```python
from build123d import *

# Parameters (mm, degrees)
SKETCH5_W                        = 20
SKETCH5_H                        = 45.5
SKETCH5_R                        = 0.55
ULTRASONIC_TRANSDUCER_BASE_DEPTH = 11
ULTRASONIC_PINS_CUTAWAY_DEPTH    = 3
STANDOFF_PROFILE_R               = 1.35
ULTRASONIC_STANDOFFS_DEPTH       = 2
ENCLOSURE_OUTER_LIMIT_W          = 158.6
ENCLOSURE_OUTER_LIMIT_H          = 63.3
ENCLOSURE_BASE_DEPTH             = 1.6
ENCLOSURE_FILLET_R               = 10
SKETCH9_R                        = 2.5
SKETCH9_R_2                      = 3
SKETCH9_R_3                      = 2
UNO_STANDOFFS_DEPTH              = 5.5
UNO_START                        = 1
SKETCH11_R                       = 1.5
UNO_STANDOFF_SCREW_HOLES_DEPTH   = 4.5
ENCLOSURE_WALL_DEPTH             = 27
ENCLOSURE_WALL_DEPTH_BACK        = 1.6
SKETCH13_R                       = 4
LED_RING_CABLE_HOLE_DEPTH        = 1.6
SKETCH14_R                       = 4
BUS_SCREW_POSTS_DEPTH            = 8
SKETCH15_R                       = 1.5
BUS_SCREW_HOLES_DEPTH            = 6
SKETCH16_R                       = 2
POWER_CORD_HOLE_DEPTH            = 1.6
FILLET1_R                        = 1.5
SKETCH6_R                        = 0.6
CUT_PIN_HOLES_DEPTH              = 10


with BuildPart() as part:
    # Sketch5 → Ultrasonic Transducer Base (new body)
    with BuildSketch(Plane(origin=(0, 0, 0), x_dir=(1, 0, 0), z_dir=(0, 1, 0))):
        with Locations((70, 1)):
            Rectangle(SKETCH5_W, SKETCH5_H)
        with Locations((61.4, 22.35)):
            Circle(SKETCH5_R, mode=Mode.SUBTRACT)
        with Locations((78.6, 22.35)):
            Circle(SKETCH5_R, mode=Mode.SUBTRACT)
        with Locations((78.6, -20.35)):
            Circle(SKETCH5_R, mode=Mode.SUBTRACT)
        with Locations((61.4, -20.35)):
            Circle(SKETCH5_R, mode=Mode.SUBTRACT)
    extrude(amount=ULTRASONIC_TRANSDUCER_BASE_DEPTH)

    # Sketch8 → Ultrasonic Pins Cutaway (cut)
    with BuildSketch(Plane(origin=(0, 11, 0), x_dir=(1, 0, 0), z_dir=(0, 1, 0))):
        Polygon((60, 1), (60, -6), (67, -6), (67, 8), (60, 8), align=None)
    extrude(amount=-ULTRASONIC_PINS_CUTAWAY_DEPTH, mode=Mode.SUBTRACT)

    # Standoff Profile → Ultrasonic Standoffs (add)
    with BuildSketch(Plane.XZ.offset(-11)):
        with Locations((61.4, 20.35)):
            Circle(STANDOFF_PROFILE_R)
        with Locations((78.6, 20.35)):
            Circle(STANDOFF_PROFILE_R)
        with Locations((61.4, -22.35)):
            Circle(STANDOFF_PROFILE_R)
        with Locations((78.6, -22.35)):
            Circle(STANDOFF_PROFILE_R)
    extrude(amount=-ULTRASONIC_STANDOFFS_DEPTH)

    # Enclosure Outer Limit → Enclosure Base (add)
    with BuildSketch(Plane(origin=(0, 0, 0), x_dir=(1, 0, 0), z_dir=(0, 1, 0))):
        with Locations((5, 0)):
            Rectangle(ENCLOSURE_OUTER_LIMIT_W, ENCLOSURE_OUTER_LIMIT_H)
    extrude(amount=-ENCLOSURE_BASE_DEPTH)

    # Enclosure Fillet
    enclosure_fillet_edges = [part.edges().sort_by_distance(p)[0] for p in [
        (-74.3, -0.8, -31.65),
        (84.3, -0.8, -31.65),
        (84.3, -0.8, 31.65),
        (-74.3, -0.8, 31.65),
    ]]
    fillet(enclosure_fillet_edges, radius=ENCLOSURE_FILLET_R)

    # Sketch9 → Uno Standoffs (add)
    with BuildSketch(Plane(origin=(0, 0, 0), x_dir=(1, 0, 0), z_dir=(0, 1, 0))):
        with Locations((-19, 24.05)):
            Circle(SKETCH9_R)
        with Locations((31.8, 8.85)):
            Circle(SKETCH9_R_2)
        with Locations((31.8, -19.05)):
            Circle(SKETCH9_R_2)
        with Locations((-20.3, -24.15)):
            Circle(SKETCH9_R)
        with Locations((-20.3, -9.15)):
            Circle(SKETCH9_R_3)
    extrude(amount=UNO_STANDOFFS_DEPTH)

    # Sketch11 → Uno Standoff Screw Holes (cut)
    with BuildSketch(Plane(origin=(0, 0, 0), x_dir=(1, 0, 0), z_dir=(0, 1, 0)).offset(UNO_START)):
        with Locations((-19, 24.05)):
            Circle(SKETCH11_R)
        with Locations((31.8, 8.85)):
            Circle(SKETCH11_R)
        with Locations((31.8, -19.05)):
            Circle(SKETCH11_R)
        with Locations((-20.3, -24.15)):
            Circle(SKETCH11_R)
    extrude(amount=UNO_STANDOFF_SCREW_HOLES_DEPTH, mode=Mode.SUBTRACT)

    # Sketch12 → Enclosure Wall (add, two sides)
    with BuildSketch(Plane(origin=(0, 0, 0), x_dir=(1, 0, 0), z_dir=(0, 1, 0))) as enclosure_wall_sk:
        with BuildLine():
            Line((85.9, -21.65), (85.9, 21.65))
            ThreePointArc((85.9, 21.65), (82.502438662, 29.852438662), (74.3, 33.25))
            Line((74.3, 33.25), (-64.3, 33.25))
            ThreePointArc((-64.3, 33.25), (-72.502438662, 29.852438662), (-75.9, 21.65))
            Line((-75.9, 21.65), (-75.9, -21.65))
            ThreePointArc((-75.9, -21.65), (-72.502438662, -29.852438662), (-64.3, -33.25))
            Line((-64.3, -33.25), (74.3, -33.25))
            ThreePointArc((74.3, -33.25), (82.502438662, -29.852438662), (85.9, -21.65))
        make_face()
        with BuildLine():
            Line((84.3, -21.65), (84.3, 21.65))
            ThreePointArc((84.3, 21.65), (81.371067812, 28.721067812), (74.3, 31.65))
            Line((74.3, 31.65), (-64.3, 31.65))
            ThreePointArc((-64.3, 31.65), (-71.371067812, 28.721067812), (-74.3, 21.65))
            Line((-74.3, 21.65), (-74.3, -21.65))
            ThreePointArc((-74.3, -21.65), (-71.371067812, -28.721067812), (-64.3, -31.65))
            Line((-64.3, -31.65), (74.3, -31.65))
            ThreePointArc((74.3, -31.65), (81.371067812, -28.721067812), (84.3, -21.65))
        make_face(mode=Mode.SUBTRACT)
    extrude(amount=ENCLOSURE_WALL_DEPTH)
    extrude(enclosure_wall_sk.sketch, amount=-ENCLOSURE_WALL_DEPTH_BACK)

    # Sketch13 → LED Ring Cable Hole (cut)
    with BuildSketch(Plane.ZY.offset(75.9)):
        with Locations((-0.209219048, 4)):
            Circle(SKETCH13_R)
    extrude(amount=-LED_RING_CABLE_HOLE_DEPTH, mode=Mode.SUBTRACT)

    # Sketch14 → Bus Screw Posts (add)
    with BuildSketch(Plane(origin=(0, 0, 0), x_dir=(1, 0, 0), z_dir=(0, 1, 0))):
        with Locations((-57.9, 23.65)):
            Circle(SKETCH14_R)
        with Locations((-57.9, -23.65)):
            Circle(SKETCH14_R)
    extrude(amount=BUS_SCREW_POSTS_DEPTH)

    # Sketch15 → Bus Screw Holes (cut)
    with BuildSketch(Plane(origin=(0, 8, 0), x_dir=(1, 0, 0), z_dir=(0, 1, 0))):
        with Locations((-57.9, 23.65)):
            Circle(SKETCH15_R)
        with Locations((-57.9, -23.65)):
            Circle(SKETCH15_R)
    extrude(amount=-BUS_SCREW_HOLES_DEPTH, mode=Mode.SUBTRACT)

    # Sketch16 → Power Cord Hole (cut)
    with BuildSketch(Plane(origin=(0, 0, -33.25), x_dir=(-1, 0, 0), z_dir=(0, 0, -1))):
        with Locations((40.05731821, 4.801042168)):
            Circle(SKETCH16_R)
    extrude(amount=-POWER_CORD_HOLE_DEPTH, mode=Mode.SUBTRACT)

    # Fillet1
    fillet1_edges = [part.edges().sort_by_distance(p)[0] for p in [
        (80, 5.5, 21.75),
        (60, 5.5, 21.75),
        (60, 5.5, -23.75),
        (80, 5.5, -23.75),
    ]]
    fillet(fillet1_edges, radius=FILLET1_R)

    # Sketch6 → Cut Pin Holes (cut)
    with BuildSketch(Plane(origin=(0, 11, 0), x_dir=(1, 0, 0), z_dir=(0, 1, 0))):
        with Locations((61.4, 22.35)):
            Circle(SKETCH6_R)
        with Locations((78.6, 22.35)):
            Circle(SKETCH6_R)
        with Locations((78.6, -20.35)):
            Circle(SKETCH6_R)
        with Locations((61.4, -20.35)):
            Circle(SKETCH6_R)
    extrude(amount=CUT_PIN_HOLES_DEPTH, mode=Mode.SUBTRACT)


solid = part.part
```
Source: CAD feature listing. Evaluate the final solid. Frame: model axes, mm. A direction names the side the tool comes from. Give positions to 0.01 mm unless a question says otherwise; leave off trailing zeros. Loops run counter-clockwise (first coordinate to the right, second up) from the corner with the lowest first, then second, coordinate; pieces in that order, holes last. Notation, with made-up numbers: (82.25, 84) -> (120.25, 84) arc R27 ccw to (120.25, 115) -> close; hole circle Ø11 at (41.25, -31). An arc over 180 degrees is marked (long way). Use a Markdown table: item, result. Add a question column.
(1) Section query C-C (z = 9.15). Output: boundary loops of the cut face in (x, y).
(2) Pull-direction query (X, two-part tool) for faces 1 (the face through (-61.896, 3.944, -23.826)), 2 (the face through (6, 13, -33.25)), 3 (the face through (82.412, 12.9, 29.942)); classes: +X half, -X half, draft (parallel to the pull), parting line (faces both ways), or undercut.
(3) Section query A-A (y = 9.5). Count the separate pieces of the cut face and the enclosed holes in it, then the cut area to 3 significant figures.
(4) First-contact query: pin 1 Ø9 at (x, z) = (-56.5, 24) entering from +Y; pin 2 Ø1.3 at (x, z) = (78.5, -22.5) entering from +Y; pin 3 Ø5 at (x, z) = (32.5, 20.5) entering from +Y. Flat tips, straight axial feed; report the tip coordinate or a pass-through.
(5) Section query D-D (y = 20.25). Output: boundary loops of the cut face in (x, z).
(6) Ray query, line 1 (Z direction, x = 31.8, y = 2.15); line 2 (X direction, y = 6.5, z = -6); line 3 (Z direction, x = 61.4, y = 2.5). Return the intervals inside material, ascending.
(7) Access query for faces 4 (the face through (-59.01, 5.04, 22.64)), 5 (the face through (85.9, 13, 0)). Directions: +Z, -Z, +X, -X, +Y, -Y. A direction counts if a zero-diameter tool reaches every point of the face in a straight line with its end or side. Return the directions, or none.
(8) Section query B-B (x = -1). Output: boundary loops of the cut face in (y, z), then the cut area to 3 significant figures.
Checked values:
| question | item | result |
|---|---|---|
| 1 | outline | (-75.9, -1.6) -> (85.9, -1.6) -> (85.9, 27) -> (84.3, 27) -> (84.3, 0) -> (80, 0) -> (80, 11) -> (60, 11) -> (60, 0) -> (-18.3, 0) -> (-18.3, 5.5) -> (-22.3, 5.5) -> (-22.3, 0) -> (-74.3, 0) -> (-74.3, 27) -> (-75.9, 27) -> close |
| 2 | face 1 | undercut |
| 2 | face 2 | draft |
| 2 | face 3 | +X half |
| 3 | separate pieces | 2 |
| 3 | enclosed holes | 5 |
| 3 | area | 1,500 mm^2 |
| 4 | pin 1 | y = 8 |
| 4 | pin 2 | y = 13 |
| 4 | pin 3 | y = 5.5 |
| 5 | outline | (-75.9, -21.65) arc R11.6 ccw to (-64.3, -33.25) -> (74.3, -33.25) arc R11.6 ccw to (85.9, -21.65) -> (85.9, 21.65) arc R11.6 ccw to (74.3, 33.25) -> (-64.3, 33.25) arc R11.6 ccw to (-75.9, 21.65) -> close; hole (-74.3, -21.65) arc R10 ccw to (-64.3, -31.65) -> (74.3, -31.65) arc R10 ccw to (84.3, -21.65) -> (84.3, 21.65) arc R10 ccw to (74.3, 31.65) -> (-64.3, 31.65) arc R10 ccw to (-74.3, 21.65) -> close |
| 6 | line 1 | -33.25 to -31.65, -11.85 to -10.35, -7.35 to -5.85, 16.05 to 17.55, 20.55 to 22.05, 31.65 to 33.25 |
| 6 | line 2 | -75.9 to -74.3, 60 to 80, 84.3 to 85.9 |
| 6 | line 3 | -33.25 to -31.65, -23.75 to -22.9, -21.8 to 19.8, 20.9 to 21.75, 31.65 to 33.25 |
| 7 | face 4 | +Y |
| 7 | face 5 | +Z, -Z, +X, +Y, -Y |
| 8 | outline | (-1.6, -33.25) -> (27, -33.25) -> (27, -31.65) -> (0, -31.65) -> (0, 31.65) -> (27, 31.65) -> (27, 33.25) -> (-1.6, 33.25) -> close |
| 8 | area | 193 mm^2 |
